```python
from build123d import *

# Parameters (mm, degrees)
SKETCH_1_W          = 40
SKETCH_1_H          = 24
EXTRUDE_1_DEPTH     = 2
SKETCH_4_W          = 60
SKETCH_4_H          = 20
EXTRUDE_3_DEPTH     = 2
CUT_EXTRUDE_3_DEPTH = 33.372828112
SKETCH_7_W          = 36
SKETCH_7_H          = 14
CUT_EXTRUDE_4_DEPTH = 33.372828112
FILLET_1_R          = 3
FILLET_2_R          = 0.4


with BuildPart() as part:
    # 草图1 → 凸台-拉伸1 (new body)
    with BuildSketch(Plane(origin=(0, 0, 0), x_dir=(1, 0, 0), z_dir=(0, 1, 0))):
        Rectangle(SKETCH_1_W, SKETCH_1_H)
    extrude(amount=EXTRUDE_1_DEPTH)

    # 草图4 → 凸台-拉伸3 (add)
    with BuildSketch(Plane(origin=(0, 2, 0), x_dir=(1, 0, 0), z_dir=(0, 1, 0))):
        Rectangle(SKETCH_4_W, SKETCH_4_H)
    extrude(amount=-EXTRUDE_3_DEPTH)

    # 草图6 → 切除-拉伸3 (cut, through all)
    with BuildSketch(Plane(origin=(0, 2, 0), x_dir=(1, 0, 0), z_dir=(0, 1, 0))):
        with BuildLine():
            Line((-25, 1.5), (-22.5, 1.5))
            ThreePointArc((-22.5, 1.5), (-21, 0), (-22.5, -1.5))
            Line((-22.5, -1.5), (-25, -1.5))
            ThreePointArc((-25, -1.5), (-26.5, 0), (-25, 1.5))
        make_face()
        with BuildLine():
            Line((-25, 5.5), (-22.5, 5.5))
            ThreePointArc((-22.5, 5.5), (-21, 4), (-22.5, 2.5))
            Line((-22.5, 2.5), (-25, 2.5))
            ThreePointArc((-25, 2.5), (-26.5, 4), (-25, 5.5))
        make_face()
        with BuildLine():
            Line((-25, -2.5), (-22.5, -2.5))
            ThreePointArc((-22.5, -2.5), (-21, -4), (-22.5, -5.5))
            Line((-22.5, -5.5), (-25, -5.5))
            ThreePointArc((-25, -5.5), (-26.5, -4), (-25, -2.5))
        make_face()
        with BuildLine():
            Line((25, -2.5), (22.5, -2.5))
            ThreePointArc((22.5, -2.5), (21, -4), (22.5, -5.5))
            Line((22.5, -5.5), (25, -5.5))
            ThreePointArc((25, -5.5), (26.5, -4), (25, -2.5))
        make_face()
        with BuildLine():
            Line((25, 1.5), (22.5, 1.5))
            ThreePointArc((22.5, 1.5), (21, 0), (22.5, -1.5))
            Line((22.5, -1.5), (25, -1.5))
            ThreePointArc((25, -1.5), (26.5, 0), (25, 1.5))
        make_face()
        with BuildLine():
            Line((25, 5.5), (22.5, 5.5))
            ThreePointArc((22.5, 5.5), (21, 4), (22.5, 2.5))
            Line((22.5, 2.5), (25, 2.5))
            ThreePointArc((25, 2.5), (26.5, 4), (25, 5.5))
        make_face()
    extrude(amount=-CUT_EXTRUDE_3_DEPTH, mode=Mode.SUBTRACT)

    # 草图7 → 切除-拉伸4 (cut, through all)
    with BuildSketch(Plane(origin=(0, 2, 0), x_dir=(1, 0, 0), z_dir=(0, 1, 0))):
        Rectangle(SKETCH_7_W, SKETCH_7_H)
    extrude(amount=-CUT_EXTRUDE_4_DEPTH, mode=Mode.SUBTRACT)

    # 圆角1
    fillet_1_edges = [part.edges().sort_by_distance(p)[0] for p in [
        (18, 1, -7),
        (18, 1, 7),
        (-18, 1, 7),
        (-18, 1, -7),
        (30, 1, 10),
        (-30, 1, -10),
        (30, 1, -10),
        (-30, 1, 10),
    ]]
    fillet(fillet_1_edges, radius=FILLET_1_R)

    # 圆角2
    fillet_2_edges = [part.edges().sort_by_distance(p)[0] for p in [
        (20, 1, 12),
        (-20, 1, 12),
        (-20, 1, -12),
        (20, 1, -12),
    ]]
    fillet(fillet_2_edges, radius=FILLET_2_R)


solid = part.part
```
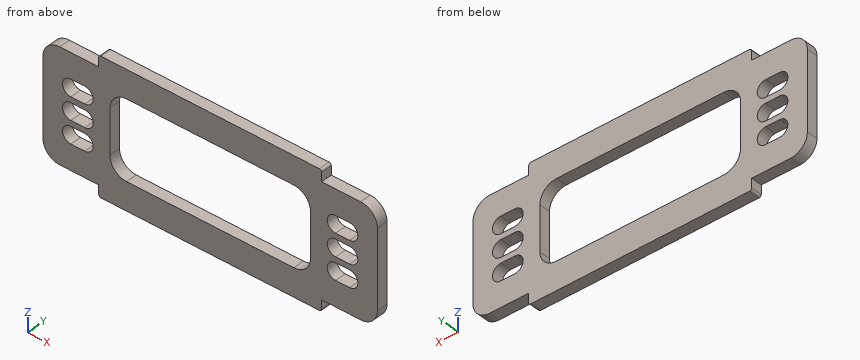
Source: CAD feature listing. Evaluate the final solid. Frame: model axes, mm. Give positions to 0.01 mm unless a question says otherwise; leave off trailing zeros. Loops run counter-clockwise (first coordinate to the right, second up) from the corner with the lowest first, then second, coordinate; pieces in that order, holes last. Notation, with made-up numbers: (45.5, 0) -> (88.5, 0) arc R9 ccw to (88.5, 6) -> close; hole circle Ø10 at (62, -18). An arc over 180 degrees is marked (long way). Use a Markdown table: item, result. Add a question column.
(1) Section query B-B (z = 0). Output: boundary loops of the cut face in (x, y), then the cut area to 3 significant figures.
(2) First-contact query: pin 1 Ø1 at (x, y) = (-24, 1) entering from +Z; pin 2 Ø0.5 at (y, z) = (0.5, 10.5) entering from -X; pin 3 Ø0.8 at (y, z) = (1, -11) entering from +X. Flat tips, straight axial feed; report the tip coordinate or a pass-through.
(3) Ray query, line 1 (Z direction, x = 24, y = 0.4); line 2 (X direction, y = 1.1, z = -4); line 3 (Z direction, x = 11, y = 1.25). Return the intervals inside material, ascending.
(4) Section query C-C (y = 0.8). Count the separate pieces of the cut face and the enclosed holes in it, then the cut area to 3 significant figures.
(5) Section query A-A (x = -1). Output: boundary loops of the cut face in (y, z).
Checked values:
| question | item | result |
|---|---|---|
| 1 | outline | (-30, 0) -> (-26.5, 0) -> (-26.5, 2) -> (-30, 2) -> close; (-21, 0) -> (-18, 0) -> (-18, 2) -> (-21, 2) -> close; (18, 0) -> (21, 0) -> (21, 2) -> (18, 2) -> close; (26.5, 0) -> (30, 0) -> (30, 2) -> (26.5, 2) -> close |
| 1 | area | 26.0 mm^2 |
| 2 | pin 1 | z = 10 |
| 2 | pin 2 | x = -20 |
| 2 | pin 3 | x = 20 |
| 3 | line 1 | -10 to -5.5, -2.5 to -1.5, 1.5 to 2.5, 5.5 to 10 |
| 3 | line 2 | -30 to -26.5, -21 to -18, 18 to 21, 26.5 to 30 |
| 3 | line 3 | -12 to -7, 7 to 12 |
| 4 | separate pieces | 1 |
| 4 | enclosed holes | 7 |
| 4 | area | 768 mm^2 |
| 5 | outline | (0, -12) -> (2, -12) -> (2, -7) -> (0, -7) -> close; (0, 7) -> (2, 7) -> (2, 12) -> (0, 12) -> close |
